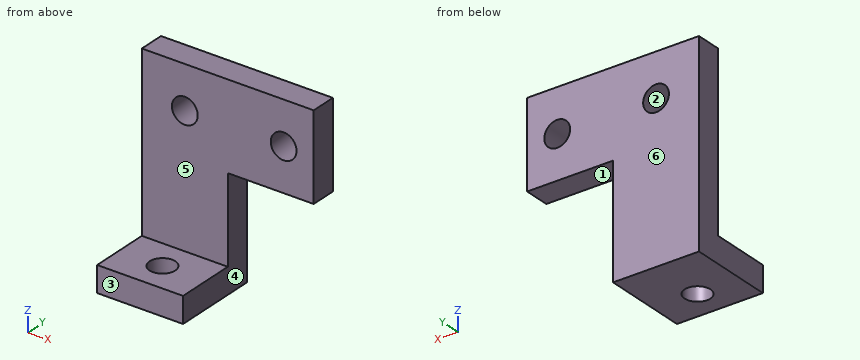
from build123d import *

# Parameters (mm, degrees)
BOSS_EXTRUDE1_DEPTH = 3
SKETCH2_W           = 10
SKETCH2_H           = 3
BOSS_EXTRUDE2_DEPTH = 10
CUT_EXTRUDE1_REACH  = 12
SKETCH3_R           = 1.5
CUT_EXTRUDE2_REACH  = 25
SKETCH4_R           = 1.5


with BuildPart() as part:
    # Sketch1 → Boss-Extrude1 (new body)
    with BuildSketch(Plane(origin=(0, 0, 0), x_dir=(1, 0, 0), z_dir=(0, 1, 0))):
        Polygon((0, 0), (0, 10), (-10, 10), (-10, -10), (10, -10), (10, 0), align=None)
    extrude(amount=BOSS_EXTRUDE1_DEPTH)

    # Sketch2 → Boss-Extrude2 (add)
    with BuildSketch(Plane(origin=(0, 3, 0), x_dir=(1, 0, 0), z_dir=(0, 1, 0))):
        with Locations((-5, 11.5)):
            Rectangle(SKETCH2_W, SKETCH2_H)
    extrude(amount=-BOSS_EXTRUDE2_DEPTH)

    # Sketch3 → Cut-Extrude1 (cut, up to next)
    with BuildSketch(Plane(origin=(0, 3, 0), x_dir=(1, 0, 0), z_dir=(0, 1, 0)), mode=Mode.PRIVATE) as cut_extrude1_sk1:
        with Locations((-5, -5)):
            Circle(SKETCH3_R)
    cut_extrude1_tool1 = extrude(cut_extrude1_sk1.sketch, amount=-CUT_EXTRUDE1_REACH, mode=Mode.PRIVATE) & part.part
    add(cut_extrude1_tool1.solids().sort_by_distance((-5, 3, 5))[0], mode=Mode.SUBTRACT)
    # Sketch3 → Cut-Extrude1 (cut, up to next)
    with BuildSketch(Plane(origin=(0, 3, 0), x_dir=(1, 0, 0), z_dir=(0, 1, 0)), mode=Mode.PRIVATE) as cut_extrude1_sk2:
        with Locations((6.5, -5)):
            Circle(SKETCH3_R)
    cut_extrude1_tool2 = extrude(cut_extrude1_sk2.sketch, amount=-CUT_EXTRUDE1_REACH, mode=Mode.PRIVATE) & part.part
    add(cut_extrude1_tool2.solids().sort_by_distance((6.5, 3, 5))[0], mode=Mode.SUBTRACT)

    # Sketch4 → Cut-Extrude2 (cut, up to next)
    with BuildSketch(Plane(origin=(0, 0, -13), x_dir=(-1, 0, 0), z_dir=(0, 0, -1)), mode=Mode.PRIVATE) as cut_extrude2_sk1:
        with Locations((5, -3.5)):
            Circle(SKETCH4_R)
    cut_extrude2_tool1 = extrude(cut_extrude2_sk1.sketch, amount=-CUT_EXTRUDE2_REACH, mode=Mode.PRIVATE) & part.part
    add(cut_extrude2_tool1.solids().sort_by_distance((-5, -3.5, -13))[0], mode=Mode.SUBTRACT)


solid = part.part
For this review, take the finished solid that the model builds, in its own axes (mm). Face numbers are marked on the shaded views. A direction names the side the tool comes from. Give positions to 0.01 mm unless a question says otherwise; leave off trailing zeros. Loops run counter-clockwise (first coordinate to the right, second up) from the corner with the lowest first, then second, coordinate; pieces in that order, holes last. Notation, with made-up numbers: M 69,26 L 124,26 A7 cw 124,30 Z; hole C 6.5,-11.5 d9. An arc over 180 degrees is marked long. Put each result on its own line as item: value. Start each with the question number.
(1) Wall thickness on L1, parallel to X at y = 1.2, z = 5; L2, parallel to Z at x = -5, y = 2.15; L3, parallel to Z at x = 6.5, y = 1.2: over which ranges is each line inside the solid? List them lowest first.
(2) Add section D-D, the plane x = 6.5. Write out the cut boundary in (y, z), then the cut area to 3 significant figures.
(3) For pin 1 (3.5 mm diameter, centred on x = -5, y = -2.5, fed in from +Z); pin 2 (2 mm diameter, centred on x = 0.5, z = -6, fed in from -Y); pin 3 (2.5 mm diameter, centred on x = 2.5, y = 2, fed in from -Z), all flat-tipped, find the tip position at first contact; note any pin that passes through.
(4) Add section A-A, the plane y = -3.5. Write out the cut boundary in (x, z).
(5) The part is to be moulded in two halves that separate along Z. For the marked faces 1, 2 and 3, say which applies: +Z half, -Z half, draft (parallel to the pull), parting line (faces both ways), or undercut.
(6) Add section C-C, the plane z = 5. Write out the cut boundary in (x, y).
(7) Add section B-B, the plane x = -5. Write out the cut boundary in (y, z).
(8) Machinability: for the marked faces 4, 5 and 6, which of the approach directions +Z, -Z, +X, -X, +Y, -Y give a long, thin tool a straight path to every point of the face, cutting with its end or side? Answer none if there is none.
Result:
1. L1: x = -10 to -6.5, -3.5 to 5, 8 to 10
1. L2: z = -13 to 3.5, 6.5 to 10
1. L3: z = 0 to 3.5, 6.5 to 10
2. outline: M 0,0 L 3,0 L 3,3.5 L 0,3.5 Z; M 0,6.5 L 3,6.5 L 3,10 L 0,10 Z
2. area: 21.0 mm^2
3. pin 1: stops at z = -10
3. pin 2: stops at y = 0
3. pin 3: stops at z = 0
4. outline: M -10,-13 L -6.5,-13 L -6.5,-10 L -10,-10 Z; M -3.5,-13 L 0,-13 L 0,-10 L -3.5,-10 Z
5. face 1: -Z half
5. face 2: undercut
5. face 3: draft
6. outline: M -10,0 L -6.5,0 L -6.5,3 L -10,3 Z; M -3.5,0 L 5,0 L 5,3 L -3.5,3 Z; M 8,0 L 10,0 L 10,3 L 8,3 Z
7. outline: M -7,-13 L -5,-13 L -5,-10 L -7,-10 Z; M -2,-13 L 3,-13 L 3,3.5 L 0,3.5 L 0,-10 L -2,-10 Z; M 0,6.5 L 3,6.5 L 3,10 L 0,10 Z
8. face 4: -Z, +X, +Y, -Y
8. face 5: +Z, +X, -X, -Y
8. face 6: +Z, -Z, +X, -X, +Y
